```python
from build123d import *

# Parameters (mm, degrees)
SKETCH_1_W          = 40
SKETCH_1_H          = 35
EXTRUDE_1_DEPTH     = 2
SKETCH_2_R          = 1.65
CUT_EXTRUDE_1_DEPTH = 2
FILLET_1_R          = 2
CUT_EXTRUDE_2_DEPTH = 10
FILLET_2_R          = 1.5


with BuildPart() as part:
    # 草图1 → 凸台-拉伸1 (new body)
    with BuildSketch(Plane.XY):
        Rectangle(SKETCH_1_W, SKETCH_1_H)
    extrude(amount=EXTRUDE_1_DEPTH)

    # 草图2 → 切除-拉伸1 (cut)
    with BuildSketch(Plane.XY.offset(2)):
        with Locations((-17, -14.5)):
            Circle(SKETCH_2_R)
        with Locations((3, -14.5)):
            Circle(SKETCH_2_R)
        with Locations((-13, -7)):
            Circle(SKETCH_2_R)
        with Locations((-13, 13)):
            Circle(SKETCH_2_R)
        with Locations((15.7, 3)):
            Circle(SKETCH_2_R)
    extrude(amount=-CUT_EXTRUDE_1_DEPTH, mode=Mode.SUBTRACT)

    # 圆角1
    fillet_1_edges = [part.edges().sort_by_distance(p)[0] for p in [
        (20, -17.5, 1),
        (-20, -17.5, 1),
        (-20, 17.5, 1),
        (20, 17.5, 1),
    ]]
    fillet(fillet_1_edges, radius=FILLET_1_R)

    # 草图3 → 切除-拉伸2 (cut)
    with BuildSketch(Plane.XY.offset(2)):
        with BuildLine():
            Line((-9, 14.65), (-9, -10.5))
            Line((-9, -10.5), (11.823480969, 1.139193668))
            ThreePointArc((11.823480969, 1.139193668), (11.400024975, 2.985344434), (11.81088684, 4.834338798))
            Line((11.81088684, 4.834338798), (-9, 14.65))
        make_face()
        with BuildLine():
            Line((-4.900820963, -10.5), (15.7, -10.5))
            Line((15.7, -10.5), (15.7, -1.3))
            ThreePointArc((15.7, -1.3), (14.334491183, -1.077423901), (13.110344983, -0.432737522))
            Line((13.110344983, -0.432737522), (-4.900820963, -10.5))
        make_face()
        with BuildLine():
            Line((-4.31166216, 14.65), (15.7, 14.65))
            Line((15.7, 14.65), (15.7, 7.3))
            ThreePointArc((15.7, 7.3), (14.334491183, 7.077423901), (13.110344983, 6.432737522))
            Line((13.110344983, 6.432737522), (-4.31166216, 14.65))
        make_face()
    extrude(amount=-CUT_EXTRUDE_2_DEPTH, mode=Mode.SUBTRACT)

    # 圆角2
    fillet_2_edges = [part.edges().sort_by_distance(p)[0] for p in [
        (-4.900820963, -10.5, 1),
        (13.110344983, -0.432737522, 1),
        (15.7, -1.3, 1),
        (15.7, -10.5, 1),
        (13.110344983, 6.432737522, 1),
        (-4.31166216, 14.65, 1),
        (15.7, 14.65, 1),
        (15.7, 7.3, 1),
        (-9, 14.65, 1),
        (11.81088684, 4.834338798, 1),
        (11.823480969, 1.139193668, 1),
        (-9, -10.5, 1),
    ]]
    fillet(fillet_2_edges, radius=FILLET_2_R)


solid = part.part
```
The listing builds one solid part. Answer for the finished solid, in the listing's coordinates (mm). A direction names the side the tool comes from. Coordinates: 2 decimals unless noted, no trailing zeros. Write each loop counter-clockwise with the first axis right and the second up, starting at its lowest first coordinate (ties: lowest second). Pieces come first, ordered by that corner, then holes. Notation, with made-up numbers: (-34, -38) -> (-21, -38) arc R17 cw to (-21, -26) -> close; hole circle Ø1 at (-0.5, 76). An arc over 180 degrees is marked (long way). Write each question's results on one line, items separated by ' | '. Start each with the question number.
1) A flat-ended cylindrical pin translates along its axis: pin 1 Ø2.5 at (x, y) = (3, -14.5) entering from -Z. Find the tip coordinate at first contact, or state that the pin passes through.
2) For a pull along Y with two mould halves and no side action, classify faces 1 (the cylindrical face through (19.4, 16.93, 1.01)), 2 (the flat face through (20, 0, 1)), 3 (the cylindrical face through (15.25, -10.07, 0.99)), 4 (the cylindrical face through (-8.278, -9.226, 0.986)) as +Y half, -Y half, draft (parallel to the pull), parting line (faces both ways), or undercut.
3) A tool of negligible diameter and unlimited length cuts with its end or side. For faces 5 (the flat face through (6.32, -4.23, 1.01)), 6 (the flat face through (-20, 0, 1)), from which of +Z, -Z, +X, -X, +Y, -Y can it reach the whole face along a straight path? Write none if from no direction.
4) A cutting plane is placed at B-B (y = -14.5). Determine the outline of the cut face in (x, z).
5) A cutting plane is placed at D-D (y = 6). Determine the outline of the cut face in (x, z).
6) Straight lines are drawn through the part: probe 1 along Y at (x, z) = (-13, 0.4); probe 2 along Y at (x, z) = (-17, 1.25); probe 3 along Y at (x, z) = (15, 1). For each, find the intervals that lie inside material, in ascending order.
7) A cutting plane is placed at C-C (x = 3). Determine the outline of the cut face in (y, z), then the cut area to 3 significant figures.
8) A cutting plane is placed at A-A (x = -17). Determine the outline of the cut face in (y, z), then the cut area to 3 significant figures.
Values follow:
1) pin 1: through
2) face 1: +Y half | face 2: draft | face 3: undercut | face 4: undercut
3) face 5: +Z, -Z | face 6: +Z, -Z, -X, +Y, -Y
4) outline: (-20, 0) -> (-18.65, 0) -> (-18.65, 2) -> (-20, 2) -> close; (-15.35, 0) -> (1.35, 0) -> (1.35, 2) -> (-15.35, 2) -> close; (4.65, 0) -> (20, 0) -> (20, 2) -> (4.65, 2) -> close
5) outline: (-20, 0) -> (-9, 0) -> (-9, 2) -> (-20, 2) -> close; (9.34, 0) -> (20, 0) -> (20, 2) -> (9.34, 2) -> close
6) probe 1: -17.5 to -8.65, -5.35 to 11.35, 14.65 to 17.5 | probe 2: -17.5 to -16.15, -12.85 to 17.5 | probe 3: -17.5 to -10.27, -1.33 to 1.51, 4.49 to 7.33, 14.42 to 17.5
7) outline: (-17.5, 0) -> (-16.15, 0) -> (-16.15, 2) -> (-17.5, 2) -> close; (-12.85, 0) -> (-10.5, 0) -> (-10.5, 2) -> (-12.85, 2) -> close; (-6.08, 0) -> (-3.79, 0) -> (-3.79, 2) -> (-6.08, 2) -> close; (8.99, 0) -> (11.2, 0) -> (11.2, 2) -> (8.99, 2) -> close; (14.65, 0) -> (17.5, 0) -> (17.5, 2) -> (14.65, 2) -> close | area: 22.1 mm²
8) outline: (-17.5, 0) -> (-16.15, 0) -> (-16.15, 2) -> (-17.5, 2) -> close; (-12.85, 0) -> (17.5, 0) -> (17.5, 2) -> (-12.85, 2) -> close | area: 63.4 mm²
